Check sheet for the drawn part. Datum: minimum x, y, z corner. Units: mm. A direction names the side the tool comes from. Coordinates: 2 decimals unless noted, no trailing zeros. Write each loop counter-clockwise with the first axis right and the second up, starting at its lowest first coordinate (ties: lowest second). Pieces come first, ordered by that corner, then holes. Notation, with made-up numbers: (83, 4) -> (109, 4) arc R31 cw to (109, 34) -> close; hole circle Ø8 at (44, 28). An arc over 180 degrees is marked (long way). Answer in a Markdown table with one row per item.
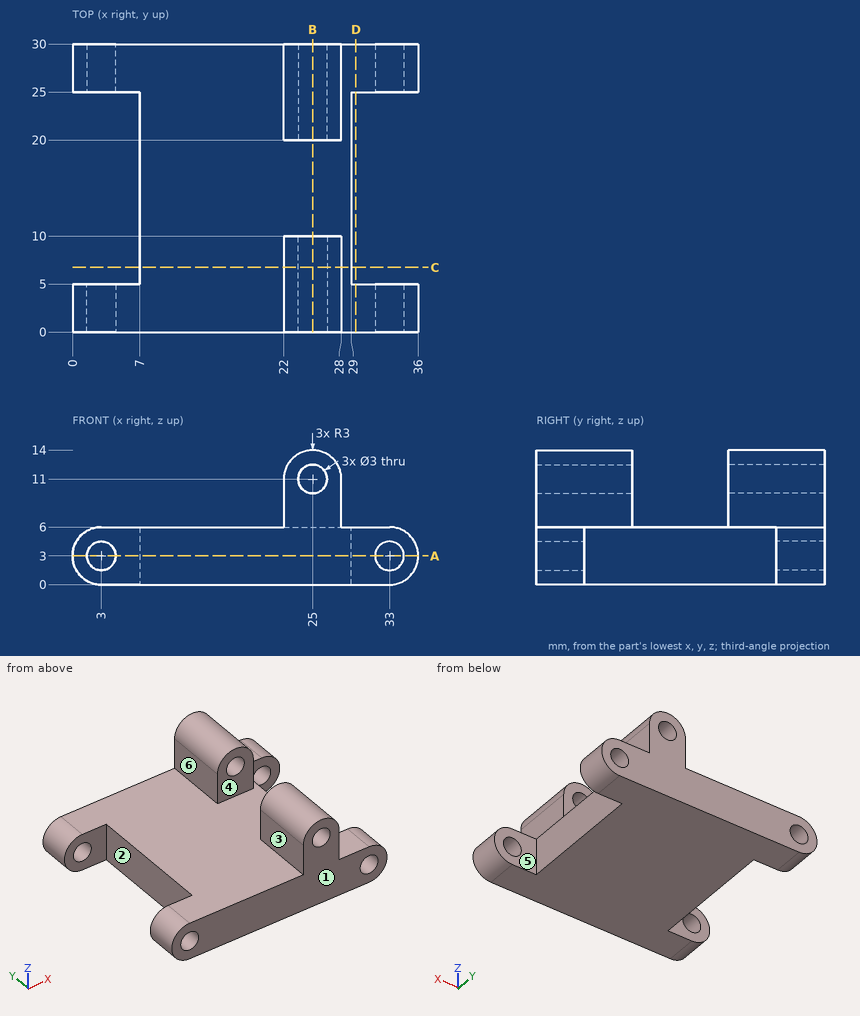
1. Sectioned sample at B-B, the plane x = 25. Record the cut outline in (y, z), and give its area (3 significant figures).
Findings below:
| item | result |
|---|---|
| outline | (0, 0) -> (30, 0) -> (30, 9.5) -> (20, 9.5) -> (20, 6) -> (10, 6) -> (10, 9.5) -> (0, 9.5) -> close; (0, 12.5) -> (10, 12.5) -> (10, 14) -> (0, 14) -> close; (20, 12.5) -> (30, 12.5) -> (30, 14) -> (20, 14) -> close |
| area | 280 mm² |
2. Release check for a two-part mould opening along Y. For the marked faces 1, 2 and 3 record: released by +Y, released by -Y, zero draft, split by the parting line, or undercut.
Findings below:
| item | result |
|---|---|
| face 1 | released by -Y |
| face 2 | undercut |
| face 3 | zero draft |
3. Material ranges on probe 1 along X at (y, z) = (1.1, 3); probe 2 along Z at (x, y) = (25, 6.5); probe 3 along X at (y, z) = (2.75, 2), recorded low to high. Write a range as from..to.
Findings below:
| item | result |
|---|---|
| probe 1 | x = 0..1.5, 4.5..31.5, 34.5..36 |
| probe 2 | z = 0..9.5, 12.5..14 |
| probe 3 | x = 0.17..1.88, 4.12..31.88, 34.12..35.83 |
4. Sectioned sample at A-A, the plane z = 3. Record the cut outline in (x, y), and give its area (3 significant figures).
Findings below:
| item | result |
|---|---|
| outline | (0, 0) -> (1.5, 0) -> (1.5, 5) -> (0, 5) -> close; (0, 25) -> (1.5, 25) -> (1.5, 30) -> (0, 30) -> close; (4.5, 0) -> (31.5, 0) -> (31.5, 5) -> (29, 5) -> (29, 25) -> (31.5, 25) -> (31.5, 30) -> (4.5, 30) -> (4.5, 25) -> (7, 25) -> (7, 5) -> (4.5, 5) -> close; (34.5, 0) -> (36, 0) -> (36, 5) -> (34.5, 5) -> close; (34.5, 25) -> (36, 25) -> (36, 30) -> (34.5, 30) -> close |
| area | 740 mm² |
5. Sectioned sample at D-D, the plane x = 29.5. Record the cut outline in (y, z), and give its area (3 significant figures).
Findings below:
| item | result |
|---|---|
| outline | (0, 0) -> (5, 0) -> (5, 6) -> (0, 6) -> close; (25, 0) -> (30, 0) -> (30, 6) -> (25, 6) -> close |
| area | 60.0 mm² |
6. Go/stop test with flat-tipped pins: pin 1 (6.5 mm diameter, centred on x = 24, z = 11, fed in from -Y); pin 2 (5 mm diameter, centred on x = 21, y = 22.5, fed in from +Z); pin 3 (8 mm diameter, centred on y = 25, z = 8.5, fed in from -X); pin 4 (9 mm diameter, centred on x = 11, y = 13.5, fed in from +Z). Record where each tip stops, or that it passes through.
Findings below:
| item | result |
|---|---|
| pin 1 | stops at y = 0 |
| pin 2 | stops at z = 13.6 |
| pin 3 | stops at x = 0.4 |
| pin 4 | stops at z = 6 |
7. Sectioned sample at C-C, the plane y = 6.75. Record the cut outline in (x, z).
Findings below:
| item | result |
|---|---|
| outline | (7, 0) -> (29, 0) -> (29, 6) -> (28, 6) -> (28, 11) arc R3 ccw to (22, 11) -> (22, 6) -> (7, 6) -> close; hole circle Ø3 at (25, 11) |
8. Access from +Z, -Z, +X, -X, +Y, -Y to the whole of each face (thin tool, end or side, straight path). Record for the marked faces 4, 5 and 6.
Findings below:
| item | result |
|---|---|
| face 4 | +Z, +X, -X |
| face 5 | +Z, -Z, +X |
| face 6 | +Z, -X, +Y, -Y |
